Work out the finished part from the listing and answer in its coordinate system (mm). A direction names the side the tool comes from. Give positions to 0.01 mm unless a question says otherwise; leave off trailing zeros. Loops run counter-clockwise (first coordinate to the right, second up) from the corner with the lowest first, then second, coordinate; pieces in that order, holes last. Notation, with made-up numbers: (-38.75, 55) - (-9.75, 55) arc R20 ccw to (-9.75, 81) - close; hole circle Ø10 at (-27, 41.5). An arc over 180 degrees is marked (long way). One line per question, with ' | ' between items. Start each with the question number.
1. Section A-A (z = 10.5) is taken. Determine the outline of the cut face in (x, y), plus the area to 3 significant figures.
2. Each of these flat-tipped pins is pushed along its axis until it touches: pin 1 (2 mm diameter, centred on x = 18, z = 19, fed in from +Y); pin 2 (2.5 mm diameter, centred on x = 11, z = 52, fed in from +Y); pin 3 (12 mm diameter, centred on x = 54.5, y = 16, fed in from -Z); pin 4 (4 mm diameter, centred on y = 15.5, z = 58.5, fed in from +X). Where does it stop, or does it pass through?
3. Section B-B (z = 41.5) is taken. Determine the outline of the cut face in (x, y).
4. Which of the six approach directions +Z, -Z, +X, -X, +Y, -Y give full straight-line access (tool end or side, diameter ignored) to faces 4 (the face through (81.837, 48.197, 34.58)), 5 (the face through (11, 18.319, 13)), 6 (the face through (70.19, 35.4, 34.51))?
5. Find the intervals of material crossed by line 1 (Y direction, x = 16, z = 50.5); line 2 (Y direction, x = 59, z = 45.5); line 3 (Y direction, x = 49, z = 17.5), in increasing order.
6. For a pull along Y with two mould halves and no side action, classify faces 1 (the face through (59, 9.425, 35)), 2 (the face through (80.029, 48.813, 68.496)), 3 (the face through (48, 38, 70)) as released by +Y, released by -Y, zero draft, split by the parting line, or undercut.
from build123d import *

# Parameters (mm, degrees)
F1_DEPTH     = 70
F2_R         = 5
F3_T1_DEPTH  = 94.0463660375
F3_T6_DEPTH  = 5
F3_T12_DEPTH = 100.881453585
F4_R         = 5
F5_T1_DEPTH  = 107.1682211358
F5_T3_DEPTH  = 60
F5_T8_DEPTH  = 5
F5_T14_DEPTH = 5
F7_DEPTH     = 6
F9_DEPTH     = 70.001


# Not quite as in the source:
# - a fillet or chamfer that OpenCascade refuses, or shapes differently, is made with other operations: its cross-section is extruded or revolved along the edge and cut away or added


with BuildPart() as f1:
    # F0 (on Top) → F1 (new body)
    with BuildSketch(Plane.XY):
        Polygon((8.0247101811, 18.3194985333), (0, 0), (102.2100174067, 0), (59.3825617324, 101.3203288608), (19.2590108271, 9.7228361946), (9.2590108271, 9.7228361946), (13.0247101811, 18.3194985333), align=None)
    extrude(amount=F1_DEPTH)

    # F2
    f2_edges = [f1.edges().sort_by_distance(p)[0] for p in [
        (80.79629, 50.660164, 70),
        (51.105009, 0, 70),
    ]]
    fillet(f2_edges, radius=F2_R)

    # F3: fillet of radius 5 on 2 edges, made by hand

    # F3_s2 → F3_t1 (cut)
    with BuildSketch(Plane.XY.offset(-29.0463660375)):
        with BuildLine():
            ThreePointArc((63.9061324741, 90.6185566458), (59.3330372536, 93.6717493047), (54.7207883471, 90.6780316604))
            Line((54.7207883471, 90.6780316604), (59.3825617324, 101.3203288608))
            Line((59.3825617324, 101.3203288608), (63.9061324741, 90.6185566458))
        make_face()
    extrude(amount=F3_T1_DEPTH, mode=Mode.SUBTRACT)


with BuildPart() as f3_tool4:
    # F3_s5 → F3_t6 (new body)
    with BuildSketch(Plane.XY.offset(65)):
        Polygon((59.3006629805, 88.6718541152), (63.9061324741, 90.6185566458), (59.3825617324, 101.3203288608), (54.7207883471, 90.6780316604), align=None)
    extrude(amount=F3_T6_DEPTH)

    # F3_s7 → F3_t8 (revolve, cut)
    with BuildSketch(Plane(origin=(59.3006629805, 88.6718541152, 65), x_dir=(-0.0064748546, -0.9999790379, 0), z_dir=(-0.9999790379, 0.0064748546, 0))):
        with BuildLine():
            ThreePointArc((0, -5), (5, 0), (0, 5))
            Line((0, 5), (0, -5))
        make_face()
    revolve(axis=Axis((59.3006629805, 88.6718541152, 65), (0, 0, 1)), mode=Mode.SUBTRACT)


with BuildPart() as f1_1:
    add(f1.part)

    # F3_t3: cut F3_tool4
    add(f3_tool4.part, mode=Mode.SUBTRACT)


with BuildPart() as f3_tool10:
    # F3_s11 → F3_t12 (new body)
    with BuildSketch(Plane(origin=(42.135637353, 96.1908566501, 0), x_dir=(0, 0, 1), z_dir=(-0.4012355091, -0.9159749267, 0))):
        with BuildLine():
            ThreePointArc((70, -18.7396238999), (68.5355339059, -15.204089994), (65, -13.7396238999))
            Line((65, -13.7396238999), (70, -13.7396238999))
            Line((70, -13.7396238999), (70, -18.7396238999))
        make_face()
    extrude(amount=F3_T12_DEPTH)

    split(bisect_by=Plane.XZ.offset(-9.7228361946), keep=Keep.BOTTOM)


with BuildPart() as f1_2:
    add(f1_1.part)

    # F3_t9: cut F3_tool10
    add(f3_tool10.part, mode=Mode.SUBTRACT)

    # F4
    f4_edges = [f1_2.edges().sort_by_distance(p)[0] for p in [
        (83.058075, 45.309278, 0),
        (36.9899, 50.200434, 0),
    ]]
    fillet(f4_edges, radius=F4_R)

    # F5: fillet of radius 5 on 1 edges, made by hand

    # F5_s2 → F5_t1 (cut)
    with BuildSketch(Plane.YZ.offset(-12.5)):
        with BuildLine():
            ThreePointArc((5, 0), (1.4644660941, 1.4644660941), (0, 5))
            Line((0, 5), (0, 0))
            Line((0, 0), (5, 0))
        make_face()
    extrude(amount=F5_T1_DEPTH, mode=Mode.SUBTRACT)

    # F5_s4 → F5_t3 (cut)
    with BuildSketch(Plane.XY.offset(5)):
        with BuildLine():
            ThreePointArc((94.6682211358, 0), (98.8355651733, 2.2371674547), (99.2736906295, 6.9467025307))
            Line((99.2736906295, 6.9467025307), (102.2100174067, 0))
            Line((102.2100174067, 0), (94.6682211358, 0))
        make_face()
    extrude(amount=F5_T3_DEPTH, mode=Mode.SUBTRACT)


with BuildPart() as f5_tool6:
    # F5_s7 → F5_t8 (new body)
    with BuildSketch(Plane.XY.offset(65)):
        Polygon((94.6682211358, 5), (94.6682211358, 0), (102.2100174067, 0), (99.2736906295, 6.9467025307), align=None)
    extrude(amount=F5_T8_DEPTH)

    # F5_s9 → F5_t10 (revolve, cut)
    with BuildSketch(Plane(origin=(94.6682211358, 5, 65), x_dir=(-0.8334688075, 0.5525665091, 0), z_dir=(0.5525665091, 0.8334688075, 0))):
        with BuildLine():
            ThreePointArc((0, -5), (5, 0), (0, 5))
            Line((0, 5), (0, -5))
        make_face()
    revolve(axis=Axis((94.6682211358, 5, 65), (0, 0, 1)), mode=Mode.SUBTRACT)


with BuildPart() as f1_3:
    add(f1_2.part)

    # F5_t5: cut F5_tool6
    add(f5_tool6.part, mode=Mode.SUBTRACT)


with BuildPart() as f5_tool12:
    # F5_s13 → F5_t14 (new body)
    with BuildSketch(Plane.XY.offset(5)):
        Polygon((94.6682211358, 5), (99.2736906295, 6.9467025307), (102.2100174067, 0), (94.6682211358, 0), align=None)
    extrude(amount=-F5_T14_DEPTH)

    # F5_s15 → F5_t16 (revolve, cut)
    with BuildSketch(Plane(origin=(94.6682211358, 5, 5), x_dir=(-0.8334688075, 0.5525665091, 0), z_dir=(-0.5525665091, -0.8334688075, 0))):
        with BuildLine():
            ThreePointArc((0, -5), (5, 0), (0, 5))
            Line((0, 5), (0, -5))
        make_face()
    revolve(axis=Axis((94.6682211358, 5, 5), (0, 0, -1)), mode=Mode.SUBTRACT)


with BuildPart() as f1_4:
    add(f1_3.part)

    # F5_t11: cut F5_tool12
    add(f5_tool12.part, mode=Mode.SUBTRACT)

    # F6 (on face) → F7 (cut)
    with BuildSketch(Plane(origin=(0, 0, 0), x_dir=(-0.4012355091, -0.9159749267, 0), z_dir=(-0.9159749267, 0.4012355091, 0))):
        with BuildLine():
            ThreePointArc((-20, 26.7366848613), (-14.1569538303, 29.1569538303), (-11.7366848613, 35))
            ThreePointArc((-11.7366848613, 35), (-14.1569538303, 40.8430461697), (-20, 43.2633151387))
            Line((-20, 43.2633151387), (-20, 26.7366848613))
        make_face()
        with BuildLine():
            Line((-20, 26.7366848613), (-20, 43.2633151387))
            ThreePointArc((-20, 43.2633151387), (-28.2633151387, 35), (-20, 26.7366848613))
        make_face()
    extrude(amount=-F7_DEPTH, mode=Mode.SUBTRACT)

    # F8 (on face) → F9 (cut, through all)
    with BuildSketch(Plane(origin=(0, 0, 0), x_dir=(1, 0, 0), z_dir=(0, 0, -1))):
        Polygon((81.168283108, -9.4247354642), (37.0782896005, -9.4247354642), (59.5163869294, -60.6483537421), align=None)
    extrude(amount=-F9_DEPTH, mode=Mode.SUBTRACT)


solid = f1_4.part
Conclusion:
1) outline: (0, 0) - (94.67, 0) arc R5 ccw to (99.27, 6.95) - (63.91, 90.62) arc R5 ccw to (54.72, 90.68) - (19.26, 9.72) - (9.26, 9.72) - (13.02, 18.32) - (8.02, 18.32) - close; hole (37.08, 9.42) - (81.17, 9.42) - (59.52, 60.65) - close | area: 3,440 mm²
2) pin 1: y = 9.72 | pin 2: y = 18.32 | pin 3: through | pin 4: x = 96.5
3) outline: (0, 0) - (94.67, 0) arc R5 ccw to (99.27, 6.95) - (63.91, 90.62) arc R5 ccw to (54.72, 90.68) - (19.26, 9.72) - (9.26, 9.72) - (10.17, 11.81) - (5.98, 13.65) - close; hole (37.08, 9.42) - (81.17, 9.42) - (59.52, 60.65) - close
4) face 4: +Z, -Z, +X, +Y | face 5: +Z, -Z, -X, +Y | face 6: +Z, -Z
5) line 1: 0 to 9.72 | line 2: 0 to 9.42, 59.47 to 93.66 | line 3: 0 to 9.42, 36.64 to 77.62
6) face 1: undercut | face 2: released by +Y | face 3: zero draft
